Geometry: see drawing. Coordinates: mm, zero at the bounding-box minimum. A direction names the side the tool comes from. Coordinates: 2 decimals unless noted, no trailing zeros. Order: outer loops, then holes, each group sorted by start corner. A loop starts at its lowest first (then second) coordinate and runs counter-clockwise, first axis right, second up. Notation, with made-up numbers: (3, 76) - (59, 76) arc R14 ccw to (59, 83) - close; hole circle Ø3 at (-37.5, 10). An arc over 180 degrees is marked (long way). Use a Markdown table: item, result. Add a question column.
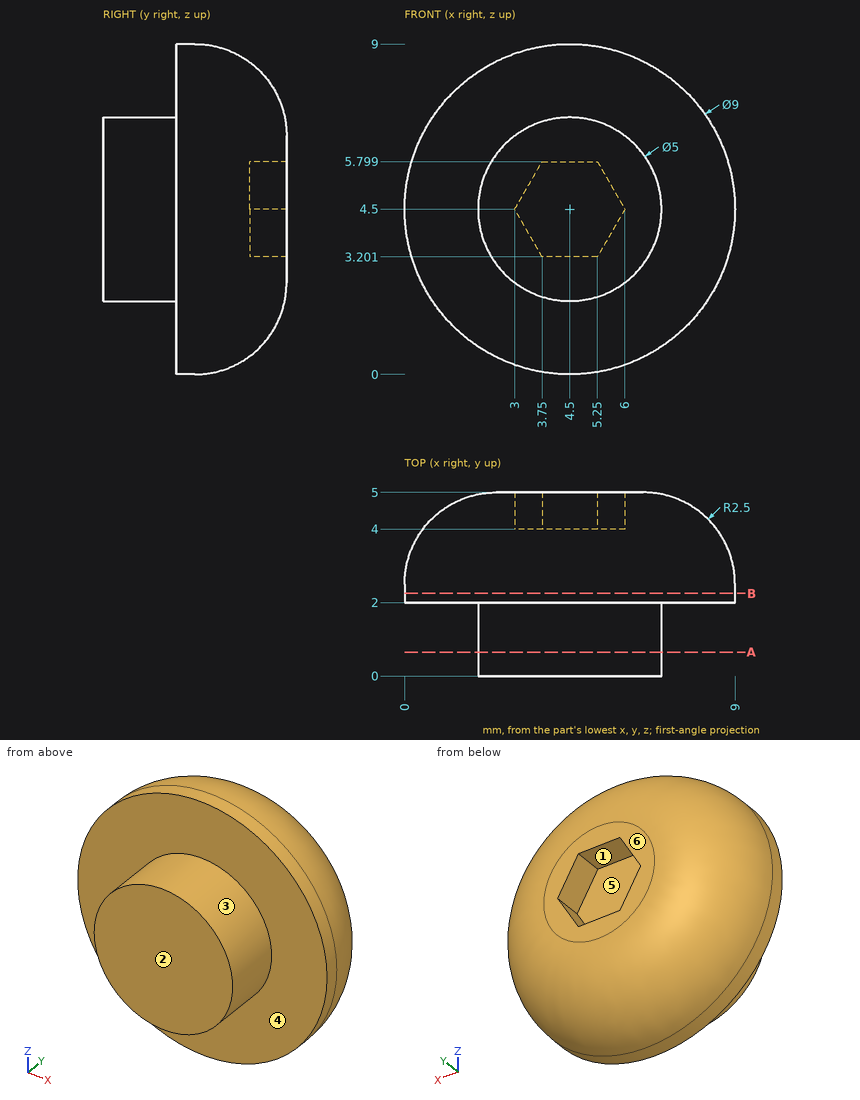
1) Access query for the marked faces 4, 5 and 6. Directions: +Z, -Z, +X, -X, +Y, -Y. A direction counts if a zero-diameter tool reaches every point of the face in a straight line with its end or side. Return the directions, or none.
2) Draft query along X for the marked faces 1, 2 and 3. Return one class per face: released by +X, released by -X, zero draft, split by the parting line, or undercut.
3) First-contact query: pin 1 (1.5 mm diameter, centred on x = 2.5, y = 4, fed in from +Z); pin 2 (3 mm diameter, centred on y = 3.5, z = 6.5, fed in from -X); pin 3 (1.3 mm diameter, centred on x = 4.5, z = 4, fed in from +Y). Flat tips, straight axial feed; report the tip coordinate or a pass-through.
4) Section query A-A (y = 0.65). Return the cut outline in (x, z).
5) Section query B-B (y = 2.25). Return the cut outline in (x, z).
6) Line query: line 1 (Y direction, x = 4.5, z = 5.5); line 2 (Z direction, x = 7.5, y = 3.9); line 3 (X direction, y = 2.75, z = 5.75). Output: solid intervals per line, ascending. Write a range as from..to.
From the geometry:
| question | item | result |
|---|---|---|
| 1 | face 4 | -Y |
| 1 | face 5 | +Y |
| 1 | face 6 | +Z, -Z, +X, -X, +Y |
| 2 | face 1 | undercut |
| 2 | face 2 | zero draft |
| 2 | face 3 | split by the parting line |
| 3 | pin 1 | stops at z = 8.55 |
| 3 | pin 2 | stops at x = 0.07 |
| 3 | pin 3 | stops at y = 4 |
| 4 | outline | circle Ø5 at (4.5, 4.5) |
| 5 | outline | circle Ø9 at (4.5, 4.5) |
| 6 | line 1 | y = 0..4 |
| 6 | line 2 | z = 1.75..7.25 |
| 6 | line 3 | x = 0.19..8.81 |
